Can you work these out from the model? Positions are in its coordinate system, mm. A direction names the side the tool comes from. Round coordinates to 2 decimals unless told otherwise and drop trailing zeros. Loops run counter-clockwise (first coordinate to the right, second up) from the corner with the lowest first, then second, coordinate; pieces in that order, holes last. Notation, with made-up numbers: M -4,75.5 L 31,75.5 A33 ccw 31,114.5 Z; hole C 19,5.25 d10. An arc over 180 degrees is marked long. Answer as CSV lines item,"result".
from build123d import *

# Parameters (mm, degrees)
F0_W     = 4.7
F0_H     = 3
F0_W_2   = 14
F2_W     = 10
F2_H     = 4.175300472
F3_DEPTH = 12.5
F5_D     = 4.4
F5_DEPTH = 14
F5_TIP   = 1.3218933619
F7_D     = 4.4
F7_DEPTH = 14
F7_TIP   = 1.3218933619
F8_SIZE  = 0.5


with BuildPart() as f1:
    # F0 (on Top) → F1 (revolve)
    with BuildSketch(Plane.XY):
        with Locations((-32.75, 1.5)):
            Rectangle(F0_W, F0_H)
        Polygon((30.4, 3), (30.4, 4), (-30.4, 4), (-30.4, 3), (-30.4, 0), (30.4, 0), align=None)
        with Locations((37.4, 1.5)):
            Rectangle(F0_W_2, F0_H)
    revolve(axis=Axis((3.1452495605, 0, 0), (1, 0, 0)))

    # F2 (on Front) → F3 (cut, symmetric)
    with BuildSketch(Plane.XZ):
        with Locations((0.4, 4.587650236)):
            Rectangle(F2_W, F2_H)
        with Locations((0.4, -4.587650236)):
            Rectangle(F2_W, F2_H)
    extrude(amount=F3_DEPTH, both=True, mode=Mode.SUBTRACT)

    # F5
    with Locations(Plane.YZ.offset(44.4)):
        with Locations((0, 0)):
            Hole(F5_D / 2, depth=F5_DEPTH)
            with Locations((0, 0, -(F5_DEPTH + F5_TIP / 2))):  # 118° drill point
                Cone(0, F5_D / 2, F5_TIP, mode=Mode.SUBTRACT)

    # F7
    with Locations(Plane(origin=(-35.1, 0, 0), x_dir=(0, -1, 0), z_dir=(-1, 0, 0))):
        with Locations((0, 0)):
            Hole(F7_D / 2, depth=F7_DEPTH)
            with Locations((0, 0, -(F7_DEPTH + F7_TIP / 2))):  # 118° drill point
                Cone(0, F7_D / 2, F7_TIP, mode=Mode.SUBTRACT)

    # F8
    f8_edges = [f1.edges().sort_by_distance(p)[0] for p in [
        (-35.1, -3, 0),
        (44.4, -3, 0),
    ]]
    chamfer(f8_edges, length=F8_SIZE)


solid = f1.part
Item 1: If we section it at B-B on x = -25: Write out the boundary of the cut face in (y, z), then the cut area to 3 significant figures.
Output:
outline,"C 0,0 d8; hole C 0,0 d4.4"
area,"35.1 mm2"
Item 2: If we section it at C-C on x = 36: Write out the boundary of the cut face in (y, z).
Output:
outline,"C 0,0 d6; hole C 0,0 d4.4"
Item 3: Will these pins go through, and if not, where does the flat tip stop? pin 1 (1.6 mm diameter, centred on y = 1, z = 3.5, fed in from -X); pin 2 (1 mm diameter, centred on x = -15.5, z = 0.5, fed in from +Y); pin 3 (3.5 mm diameter, centred on y = 0, z = 0, fed in from -X); pin 4 (1.2 mm diameter, centred on y = 1, z = -3, fed in from -X).
Output:
pin 1,"stops at x = -34.76"
pin 2,"stops at y = 4"
pin 3,"stops at x = -20.83"
pin 4,"stops at x = -35.04"
Item 4: We'd pull the mould along X, two halves only. Please class faces 5 (the face through (0, 0, -2.5)), 6 (the face through (-20.008, 0.083, -0.373)), 7 (the face through (-32, -3, 0)), 8 (the face through (30.4, -1, 3)): released by +X, released by -X, zero draft, split by the parting line, or undercut.
Output:
face 5,"undercut"
face 6,"released by -X"
face 7,"zero draft"
face 8,"released by +X"
Item 5: On a 3-axis mill with a long thin cutter (end or side, diameter ignored), from which of +Z, -Z, +X, -X, +Y, -Y can I reach the whole of each face in a straight line? I mean faces 1 (the face through (0, 0, 2.5)), 2 (the face through (5.4, 0, -3)), 3 (the face through (-30.4, 1, 3)), 4 (the face through (37, -3, 0)). Say none if no direction works.
Output:
face 1,"+Z, +Y, -Y"
face 2,"-Z, +Y, -Y"
face 3,"-X"
face 4,"+X"
Item 6: If we section it at A-A on x = 17: Write out the boundary of the cut face in (y, z).
Output:
outline,"C 0,0 d8"
Item 7: If I drill on line 1 along Z through (x, y) = (33.5, 0); line 2 along Z through (x, y) = (-27.5, 0); line 3 along X through (y, z) = (-0.5, -3.25), over which ranges is the centre line in solid material (lowest first)? Write a range as from..to.
Output:
line 1,"z = -3..-2.2, 2.2..3"
line 2,"z = -4..-2.2, 2.2..4"
line 3,"x = -30.4..-4.6, 5.4..30.4"
